Verification items for the finished model (mm, model axes). A direction names the side the tool comes from. Coordinates: 2 decimals unless noted, no trailing zeros. Loops run counter-clockwise (first coordinate to the right, second up) from the corner with the lowest first, then second, coordinate; pieces in that order, holes last.
Q1. Sectioned sample at B-B (x = 31). Enter the section's corners in (y, z).
Q2. Sectioned sample at A-A (z = 0). Enter the section's corners in (x, y).
Q3. Sectioned sample at D-D (x = 0). Enter the section's corners in (y, z), then the cut area to 4 significant figures.
Q4. Material ranges on probe 1 along Y at (x, z) = (31, -4); probe 2 along X at (y, z) = (3.75, 0.25); probe 3 along Z at (x, y) = (33, 3.5), recorded low to high.
Q5. Access from +Z, -Z, +X, -X, +Y, -Y to the whole of each face (thin tool, end or side, straight path). Record for faces 1 (the face through (18.6, -0.1, -2.43)), 2 (the face through (21, 0, -7.5)), 3 (the face through (21, 0, 7.5)).
Q6. Go/stop test with flat-tipped pins: P1, Ø4, axis at x = 28.5, y = 0.5, coming from the -Z side; P2, Ø1.5, axis at y = -1.5, z = -3, coming from the -X side; P3, Ø5.5, axis at x = 31, y = -0.27, coming from the -Z side; P4, Ø0.6, axis at y = -1.5, z = 0, coming from the +X side. Record where each tip stops, or that it passes through.
Q7. Mould release check, pull along Y, two halves, no side actions. Record for faces 4 (the face through (-8.635, -7.365, -0.119)), 5 (the face through (28.003, -0.135, -4.972)), 6 (the face through (18.57, 0.1, 2.4)): +Y half, -Y half, draft (parallel to the pull), parting line (faces both ways), or undercut.
Q8. Sectioned sample at C-C (y = -4.5). Enter the section's corners in (x, z), then the cut area to 3 significant figures.
```python
from build123d import *

# Parameters (mm, degrees)
SKETCH1_R           = 9
SKETCH1_R_2         = 4
BOSS_EXTRUDE1_DEPTH = 7.5
SKETCH2_W           = 32
SKETCH2_H           = 15
BOSS_EXTRUDE2_DEPTH = 7.5
SKETCH3_W           = 38
SKETCH3_H           = 6
CUT_EXTRUDE1_DEPTH  = 19
SKETCH4_R           = 3
CUT_EXTRUDE2_DEPTH  = 22
FILLET1_R           = 2
FILLET2_R           = 1
CHAMFER1_SIZE       = 0.5
CHAMFER2_SIZE       = 0.5
CHAMFER3_SIZE       = 0.5
FILLET3_R           = 10


with BuildPart() as part:
    # Sketch1 → Boss-Extrude1 (new, symmetric)
    with BuildSketch(Plane(origin=(0, 0, 0), x_dir=(1, 0, 0), z_dir=(0, 1, 0))):
        with Locations(Location((0, 0, 0), (0, 0, 270))):
            Circle(SKETCH1_R)
        with Locations(Location((0, 0, 0), (0, 0, 270))):
            Circle(SKETCH1_R_2, mode=Mode.SUBTRACT)
    extrude(amount=BOSS_EXTRUDE1_DEPTH, both=True)

    # Sketch2 → Boss-Extrude2 (add, symmetric)
    with BuildSketch(Plane(origin=(0, 0, 0), x_dir=(1, 0, 0), z_dir=(0, 1, 0))):
        with Locations((21, 0)):
            Rectangle(SKETCH2_W, SKETCH2_H)
    extrude(amount=BOSS_EXTRUDE2_DEPTH, both=True)

    # Sketch3 → Cut-Extrude1 (cut, symmetric)
    with BuildSketch(Plane(origin=(0, 0, 0), x_dir=(1, 0, 0), z_dir=(0, 1, 0))):
        with Locations((37, 0)):
            Rectangle(SKETCH3_W, SKETCH3_H)
    extrude(amount=CUT_EXTRUDE1_DEPTH, both=True, mode=Mode.SUBTRACT)

    # Sketch4 → Cut-Extrude2 (cut, symmetric)
    with BuildSketch(Plane.XY.offset(-3)):
        with Locations((31, -0.267092661)):
            Circle(SKETCH4_R)
    extrude(amount=CUT_EXTRUDE2_DEPTH, both=True, mode=Mode.SUBTRACT)

    # Fillet1
    fillet1_edges = [part.edges().sort_by_distance(p)[0] for p in [
        (18, 0, 3),
        (18, 0, -3),
    ]]
    fillet(fillet1_edges, radius=FILLET1_R)

    # Fillet2
    fillet2_edges = [part.edges().sort_by_distance(p)[0] for p in [
        (37, 0, 7.5),
        (37, 0, -7.5),
        (37, 0, -3),
        (37, 0, 3),
    ]]
    fillet(fillet2_edges, radius=FILLET2_R)

    # Chamfer1
    chamfer1_edges = [part.edges().sort_by_distance(p)[0] for p in [
        (28, -0.267092661, 7.5),
        (28, -0.267092661, -7.5),
        (0, -7.5, -4),
        (0, 7.5, -4),
    ]]
    chamfer(chamfer1_edges, length=CHAMFER1_SIZE)

    # Chamfer2
    chamfer2_edges = [part.edges().sort_by_distance(p)[0] for p in [
        (20.5, 7.5, -7.5),
        (20.5, -7.5, -7.5),
        (36.707106781, -7.5, -7.207106781),
        (37, -7.5, -5.25),
        (37, 7.5, -5.25),
        (36.707106781, -7.5, -3.292893219),
        (28, -7.5, -3),
        (18.585786438, -7.5, -2.414213562),
        (18, -7.5, 0),
        (18.585786438, -7.5, 2.414213562),
        (28, -7.5, 3),
        (36.707106781, -7.5, 3.292893219),
        (37, -7.5, 5.25),
        (37, 7.5, 5.25),
        (36.707106781, -7.5, 7.207106781),
        (20.5, -7.5, 7.5),
        (20.5, 7.5, 7.5),
        (36.707106781, 7.5, -7.207106781),
        (36.707106781, 7.5, -3.292893219),
        (28, 7.5, -3),
        (18.585786438, 7.5, -2.414213562),
        (18, 7.5, 0),
        (18.585786438, 7.5, 2.414213562),
        (28, 7.5, 3),
        (36.707106781, 7.5, 3.292893219),
        (36.707106781, 7.5, 7.207106781),
    ]]
    chamfer(chamfer2_edges, length=CHAMFER2_SIZE)

    # Chamfer3
    chamfer3_edges = [part.edges().sort_by_distance(p)[0] for p in [
        (-9, 7.5, 0),
        (-9, -7.5, 0),
    ]]
    chamfer(chamfer3_edges, length=CHAMFER3_SIZE)

    # Fillet3
    # the kernel refuses this fillet: 10 mm, written as the material it takes off along each edge
    with BuildSketch(Plane(origin=(5, 8.443576575, -7.5), x_dir=(0, 0, 1), z_dir=(0, -1, 0))) as fillet3_piece_1:
        with BuildLine():
            CenterArc((10, -0.57743063), FILLET3_R, 176.6897249, 3.3102751)
            Line((0, -0.57743063), (0, 0))
            Line((0, 0), (0.016685226, 0))
        make_face()
    extrude(amount=16.887153149, mode=Mode.SUBTRACT)
    with BuildSketch(Plane(origin=(5, 8.443576575, 7.5), x_dir=(0, 0, -1), z_dir=(0, -1, 0))) as fillet3_piece_2:
        with BuildLine():
            CenterArc((10, 0.57743063), FILLET3_R, 180, 3.3102751)
            Line((0, 0.57743063), (0, 0))
            Line((0, 0), (0.016685226, 0))
        make_face()
    extrude(amount=16.887153149, mode=Mode.SUBTRACT)


solid = part.part
```
Geometry check:
1. outline: (-7.5, -7) - (-7, -7.5) - (-3.77, -7.5) - (-3.27, -7) - (-3.27, -3) - (-7, -3) - (-7.5, -3.5) - close; (-7.5, 3.5) - (-7, 3) - (-3.27, 3) - (-3.27, 7) - (-3.77, 7.5) - (-7, 7.5) - (-7.5, 7) - close; (2.73, -7) - (3.23, -7.5) - (7, -7.5) - (7.5, -7) - (7.5, -3.5) - (7, -3) - (2.73, -3) - close; (2.73, 3) - (7, 3) - (7.5, 3.5) - (7.5, 7) - (7, 7.5) - (3.23, 7.5) - (2.73, 7) - close
2. outline: (-9, -7) - (-8.5, -7.5) - (-4.5, -7.5) - (-4, -7) - (-4, 7) - (-4.5, 7.5) - (-8.5, 7.5) - (-9, 7) - close; (4, -7) - (4.5, -7.5) - (17.5, -7.5) - (18, -7) - (18, 7) - (17.5, 7.5) - (4.5, 7.5) - (4, 7) - close
3. outline: (-7.5, -7) - (-5.5, -9) - (5.5, -9) - (7.5, -7) - (7.5, -4.5) - (7, -4) - (-7, -4) - (-7.5, -4.5) - close; (-7.5, 4.5) - (-7, 4) - (7, 4) - (7.5, 4.5) - (7.5, 7) - (5.5, 9) - (-5.5, 9) - (-7.5, 7) - close
3. area: 141.5 mm2
4. probe 1: y = -7.5 to -3.27, 2.73 to 7.5
4. probe 2: x = -9 to -3.99, 3.99 to 18
4. probe 3: z = -7.5 to -3, 3 to 7.5
5. face 1: +X, +Y, -Y
5. face 2: -Z, +X, +Y, -Y
5. face 3: +Z, +X, +Y, -Y
6. P1: stops at z = -7.5
6. P2: stops at x = -8.71
6. P3: passes through
6. P4: stops at x = 18
7. face 4: -Y half
7. face 5: undercut
7. face 6: draft
8. outline: (5, -7.48) arc R10 ccw to (5.58, -7.5) - (36, -7.5) arc R1 ccw to (37, -6.5) - (37, -4) arc R1 ccw to (36, -3) - (20, -3) arc R2 cw to (18, -1) - (18, 1) arc R2 cw to (20, 3) - (36, 3) arc R1 ccw to (37, 4) - (37, 6.5) arc R1 ccw to (36, 7.5) - (5.58, 7.5) arc R10 ccw to (5, 7.48) arc R9 ccw (long way) to start; hole circle Ø8 at (0, 0)
8. area: 529 mm2
